from build123d import *
from OCP.BRepFilletAPI import BRepFilletAPI_MakeChamfer

# Parameters (mm, degrees)
SKETCH1_W           = 65
SKETCH1_H           = 64
SKETCH1_W_2         = 44.2
SKETCH1_H_2         = 40
BOSS_EXTRUDE1_DEPTH = 15
SKETCH3_W           = 7
SKETCH3_H           = 11.1
SKETCH4_R           = 9.5
CUT_EXTRUDE2_DEPTH  = 74.986485252
SKETCH5_R           = 4
CUT_EXTRUDE3_DEPTH  = 74.32973476
SKETCH8_R           = 2.15
CUT_EXTRUDE6_DEPTH  = 49.013019068
FILLET1_R           = 20
CHAMFER1_SIZE       = 3
CHAMFER1_SIZE2      = 1.732050808
SKETCH9_W           = 12
SKETCH9_H           = 3
SKETCH10_W          = 24
SKETCH10_H          = 5.5
BOSS_EXTRUDE2_DEPTH = 15
BOSS_EXTRUDE3_START = 9
SKETCH12_W          = 24
SKETCH12_H          = 3.7
BOSS_EXTRUDE3_DEPTH = 6
BOSS_EXTRUDE4_DEPTH = 1.3
CHAMFER2_SIZE2      = 1.339745962
CHAMFER2_SIZE       = 5
CHAMFER3_SIZE       = 10
CHAMFER3_SIZE2      = 5.773502692


with BuildPart() as part:
    # Sketch1 → Boss-Extrude1 (new body)
    with BuildSketch(Plane(origin=(0, 0, 0), x_dir=(1, 0, 0), z_dir=(0, 1, 0))):
        Rectangle(SKETCH1_W, SKETCH1_H)
        Rectangle(SKETCH1_W_2, SKETCH1_H_2, mode=Mode.SUBTRACT)
    extrude(amount=BOSS_EXTRUDE1_DEPTH)

    # Sketch3 → Cut-Revolve1 (revolve, cut)
    with BuildSketch(Plane(origin=(0, 15, 0), x_dir=(1, 0, 0), z_dir=(0, 1, 0))):
        with Locations((25.6, -5.55)):
            Rectangle(SKETCH3_W, SKETCH3_H)
        with Locations((-25.6, -5.55)):
            Rectangle(SKETCH3_W, SKETCH3_H)
    revolve(axis=Axis((22.1, 15, 0), (1, 0, 0)), mode=Mode.SUBTRACT)

    # Sketch4 → Cut-Extrude2 (cut, through all)
    with BuildSketch(Plane(origin=(32.5, 0, 0), x_dir=(0, 0, -1), z_dir=(1, 0, 0))):
        with Locations((0, 15)):
            Circle(SKETCH4_R)
    extrude(amount=-CUT_EXTRUDE2_DEPTH, mode=Mode.SUBTRACT)

    # Sketch5 → Cut-Extrude3 (cut, through all)
    with BuildSketch(Plane.XY.offset(32)):
        with Locations((0, 15)):
            Circle(SKETCH5_R)
    extrude(amount=-CUT_EXTRUDE3_DEPTH, mode=Mode.SUBTRACT)

    # Sketch8 → Cut-Extrude6 (cut, through all)
    with BuildSketch(Plane(origin=(0, 15, 0), x_dir=(1, 0, 0), z_dir=(0, 1, 0))):
        with Locations((18, 16.5)):
            Circle(SKETCH8_R)
        with Locations((18, -16.5)):
            Circle(SKETCH8_R)
        with Locations((-18, -16.5)):
            Circle(SKETCH8_R)
        with Locations((-18, 16.5)):
            Circle(SKETCH8_R)
        with Locations(Location((9, -27, 0), (0, 0, 270))):
            Circle(SKETCH8_R)
        with Locations(Location((-9, -27, 0), (0, 0, 270))):
            Circle(SKETCH8_R)
        with Locations(Location((-9, 27, 0), (0, 0, 270))):
            Circle(SKETCH8_R)
        with Locations(Location((9, 27, 0), (0, 0, 270))):
            Circle(SKETCH8_R)
    extrude(amount=-CUT_EXTRUDE6_DEPTH, mode=Mode.SUBTRACT)

    # Fillet1
    fillet1_edges = [part.edges().sort_by_distance(p)[0] for p in [
        (-32.5, 7.5, -32),
        (32.5, 7.5, -32),
        (32.5, 7.5, 32),
        (-32.5, 7.5, 32),
    ]]
    fillet(fillet1_edges, radius=FILLET1_R)

    # Chamfer1: one chamfer whose edges measure the first distance from different faces: ONE call of the kernel's chamfer builder (chamfer() names one face for all edges)
    chamfer1_edges_1 = [part.edges().sort_by_distance(p)[0] for p in [
        (22.1, 3.9, 0),
    ]]
    chamfer1_side_1 = [part.faces().sort_by_distance(p)[0] for p in [
        (22.1, 0.427200187, 0),
    ]]
    chamfer1_edges_2 = [part.edges().sort_by_distance(p)[0] for p in [
        (-22.1, 3.9, 0),
    ]]
    chamfer1_side_2 = [part.faces().sort_by_distance(p)[0] for p in [
        (-22.1, 0.427200187, 0),
    ]]
    chamfer1 = BRepFilletAPI_MakeChamfer(part.part.solid().wrapped)
    for e in chamfer1_edges_1:
        chamfer1.Add(CHAMFER1_SIZE, CHAMFER1_SIZE2, e.wrapped, chamfer1_side_1[0].wrapped)  # the first distance lies on this face
    for e in chamfer1_edges_2:
        chamfer1.Add(CHAMFER1_SIZE, CHAMFER1_SIZE2, e.wrapped, chamfer1_side_2[0].wrapped)  # the first distance lies on this face
    add(Compound.cast(chamfer1.Shape()), mode=Mode.REPLACE)

    # Sketch9 → Cut-Revolve2 (revolve, cut)
    with BuildSketch(Plane(origin=(0, 15, 0), x_dir=(1, 0, 0), z_dir=(0, 1, 0))):
        with Locations((-6, -21.5)):
            Rectangle(SKETCH9_W, SKETCH9_H)
        with Locations((-6, 21.5)):
            Rectangle(SKETCH9_W, SKETCH9_H)
    revolve(axis=Axis((0, 15, -29.871415895), (0, 0, 1)), mode=Mode.SUBTRACT)

    # Sketch10 → Boss-Extrude2 (add)
    with BuildSketch(Plane.ZY.offset(32.5)):
        with Locations((0, 2.75)):
            Rectangle(SKETCH10_W, SKETCH10_H)
    extrude(amount=BOSS_EXTRUDE2_DEPTH)

    # Sketch12 → Boss-Extrude3 (add)
    with BuildSketch(Plane.ZY.offset(32.5).offset(BOSS_EXTRUDE3_START)):
        with Locations((0, 7.35)):
            Rectangle(SKETCH12_W, SKETCH12_H)
    extrude(amount=BOSS_EXTRUDE3_DEPTH)

    # Sketch13 → Boss-Extrude4 (add)
    with BuildSketch(Plane(origin=(0, 9.2, 0), x_dir=(1, 0, 0), z_dir=(0, 1, 0))):
        Polygon((-46.4, 2.2), (-46.4, 1.6), (-47.5, 1.6), (-47.5, 12), (-41.5, 12), (-41.5, -12), (-47.5, -12), (-47.5, -1.6), (-46.4, -1.6), (-46.4, -2.2), (-43.2, -2.2), (-43.2, 2.2), align=None)
    extrude(amount=BOSS_EXTRUDE4_DEPTH)

    # Chamfer2
    chamfer2_edges = [part.edges().sort_by_distance(p)[0] for p in [
        (-41.5, 10.5, 0),
    ]]
    chamfer2_side = [part.faces().sort_by_distance(p)[0] for p in [
        (-41.5, 10.473205081, 0),
    ]]
    chamfer(chamfer2_edges, length=CHAMFER2_SIZE - 0.0001, length2=CHAMFER2_SIZE2 - 0.0001, reference=chamfer2_side[0])  # a hair under: the kernel refuses the full size

    # Chamfer3: one chamfer whose edges measure the first distance from different faces: ONE call of the kernel's chamfer builder (chamfer() names one face for all edges)
    chamfer3_edges_1 = [part.edges().sort_by_distance(p)[0] for p in [
        (-47.5, 5.25, 12),
    ]]
    chamfer3_side_1 = [part.faces().sort_by_distance(p)[0] for p in [
        (-41.177093858, 4.00630158, 12),
    ]]
    chamfer3_edges_2 = [part.edges().sort_by_distance(p)[0] for p in [
        (-47.5, 5.25, -12),
    ]]
    chamfer3_side_2 = [part.faces().sort_by_distance(p)[0] for p in [
        (-41.177093858, 4.00630158, -12),
    ]]
    chamfer3 = BRepFilletAPI_MakeChamfer(part.part.solid().wrapped)
    for e in chamfer3_edges_1:
        chamfer3.Add(CHAMFER3_SIZE, CHAMFER3_SIZE2, e.wrapped, chamfer3_side_1[0].wrapped)  # the first distance lies on this face
    for e in chamfer3_edges_2:
        chamfer3.Add(CHAMFER3_SIZE, CHAMFER3_SIZE2, e.wrapped, chamfer3_side_2[0].wrapped)  # the first distance lies on this face
    add(Compound.cast(chamfer3.Shape()), mode=Mode.REPLACE)


solid = part.part
Source: CAD feature listing. Evaluate the final solid. Frame: model axes, mm. A direction names the side the tool comes from. Coordinates: 2 decimals unless noted, no trailing zeros. Order: outer loops, then holes, each group sorted by start corner. A loop starts at its lowest first (then second) coordinate and runs counter-clockwise, first axis right, second up. Notation, with made-up numbers: M 10.25,-33.75 L 61.25,-33.75 A11 cw 61.25,-27.75 Z; hole C -35,-24.5 d9. An arc over 180 degrees is marked long. Write each question's results on one line, items separated by ' | '. Start each with the question number.
1. Section C-C, the plane z = -17. Return the cut outline in (x, y).
2. Reachability of faces 5 (the face through (-35, 3, 12)), 6 (the face through (-22.1, 0.7, 0.3)), 7 (the face through (26.5, 3.9, 0.2)) from +Z, -Z, +X, -X, +Y, -Y: full face, straight path, thin tool, end or side. Return the list, or none.
3. Section A-A, the plane x = 0. Return the cut outline in (y, z), then the cut area to 3 significant figures.
4. Section B-B, the plane z = -27. Return the cut outline in (x, y), then the cut area to 3 significant figures.
5. Material intervals for L1, parallel to X at y = 5.25, z = 27; L2, parallel to Z at x = -7.5, y = 7.5; L3, parallel to X at y = 5.5, z = 28.5, sorted ascending.
6. Draft query along Z for faces 1 (the face through (-35, 3, -12)), 2 (the face through (0, 2, -20)), 3 (the face through (0, 7, 32)), 4 (the face through (-42.18, 8.04, -0.14)). Return one class per face: +Z half, -Z half, draft (parallel to the pull), parting line (faces both ways), or undercut.
7. Pin query (flat end, axial travel): pin 1 (1.4 mm diameter, centred on x = -44.5, y = 9.5, fed in from +Z); pin 2 (4 mm diameter, centred on x = -9, z = 27, fed in from +Y); pin 3 (2.5 mm diameter, centred on x = -35.5, y = 3.5, fed in from +Z); pin 4 (1 mm diameter, centred on x = -45.5, y = 10, fed in from -Z). Return the tip coordinate at first contact, or that it passes through.
8. Section D-D, the plane x = 9. Return the cut outline in (y, z).
Solution:
1) outline: M -31.86,0 L -22.1,0 L -22.1,15 L -31.86,15 Z; M 22.1,0 L 31.86,0 L 31.86,15 L 22.1,15 Z
2) face 5: +Z, -X, +Y, -Y | face 6: +Y, -Y | face 7: +Y
3) outline: M 0,-32 L 11,-32 L 11,-23 L 3,-23 L 3,-20 L 0,-20 Z; M 0,20 L 3,20 L 3,23 L 11,23 L 11,32 L 0,32 Z | area: 216 mm²
4) outline: M -25.73,0 L -11.15,0 L -11.15,15 L -25.73,15 Z; M -6.85,0 L 6.85,0 L 6.85,15 L 4,15 A4 cw -4,15 L -6.85,15 Z; M 11.15,0 L 25.73,0 L 25.73,15 L 11.15,15 Z | area: 618 mm²
5) L1: -25.73 to -11.15, -6.85 to 6.85, 11.15 to 25.73 | L2: -32 to -28.54, -25.46 to -23, 23 to 25.46, 28.54 to 32 | L3: -23.8 to -10.54, -7.46 to 7.46, 10.54 to 23.8
6) face 1: -Z half | face 2: undercut | face 3: +Z half | face 4: draft
7) pin 1: z = 8.36 | pin 2: through | pin 3: z = 12 | pin 4: z = -7.67
8) outline: M 0,-32 L 15,-32 L 15,-29.15 L 0,-29.15 Z; M 0,-24.85 L 15,-24.85 L 15,-23 L 7.06,-23 L 7.06,-20 L 0,-20 Z; M 0,20 L 7.06,20 L 7.06,23 L 15,23 L 15,24.85 L 0,24.85 Z; M 0,29.15 L 15,29.15 L 15,32 L 0,32 Z
